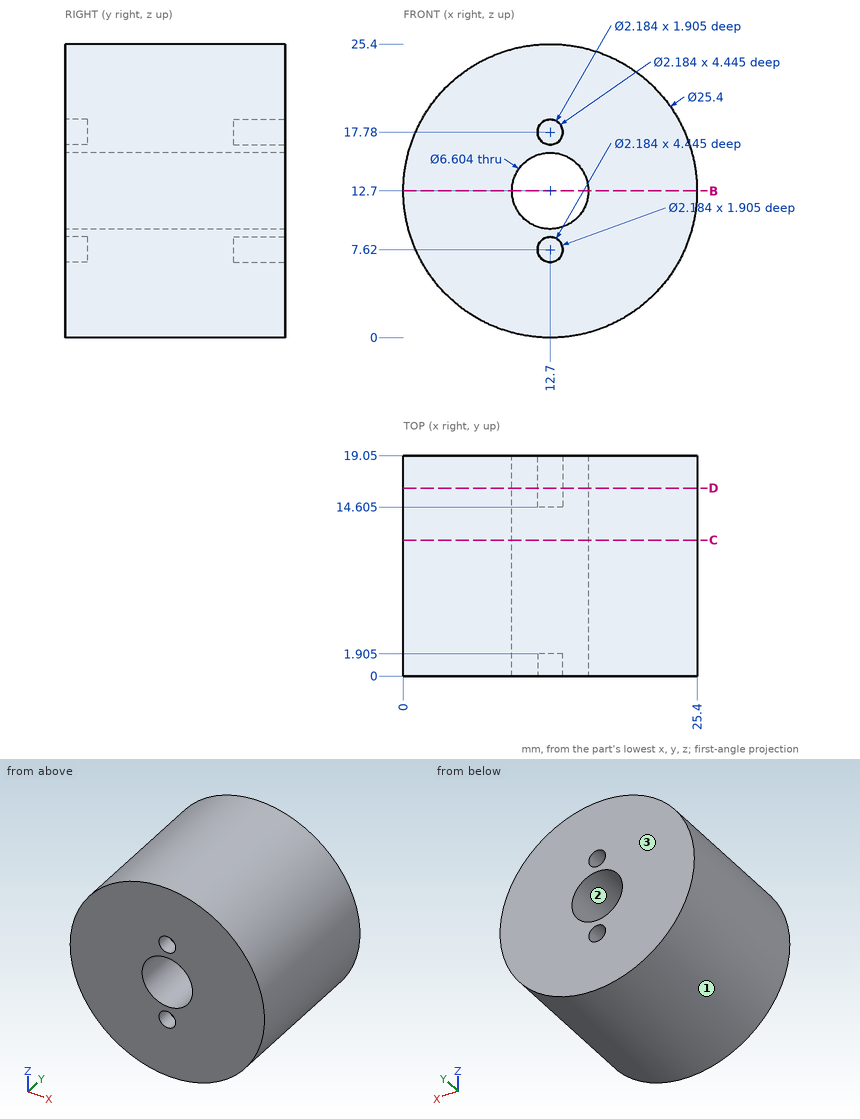
Answer from the drawing. Dimensions are ordinates in mm from the lowest x, y and z of the part. Round coordinates to 2 decimals unless told otherwise and drop trailing zeros. Loops run counter-clockwise (first coordinate to the right, second up) from the corner with the lowest first, then second, coordinate; pieces in that order, holes last. Notation, with made-up numbers: M -12,83 L 2,83 A3 cw 2,88 Z; hole C -14.5,-7 d5. An arc over 180 degrees is marked long. One line per question, with ' | ' between items. Start each with the question number.
(1) A cutting plane is placed at D-D on y = 16.25. Write down the section's boundary in (x, z) (1 decimal).
(2) Flat-ended cylindrical pins translate along their axes: pin 1 Ø0.7 at (x, z) = (13, 18) entering from +Y (3 decimals); pin 2 Ø3 at (x, z) = (4.5, 7.5) entering from -Y; pin 3 Ø10 at (x, y) = (22, 16) entering from -Z; pin 4 Ø2 at (x, z) = (12.7, 17.78) entering from -Y (3 decimals). Find the tip coordinate at first contact, or state that the pin passes through.
(3) A cutting plane is placed at C-C on y = 11.75. Write down the section's boundary in (x, z).
(4) A cutting plane is placed at B-B on z = 12.7. Write down the section's boundary in (x, y).
(5) For a pull along Z with two mould halves and no side action, classify the marked faces 1, 2 and 3 as released by +Z, released by -Z, zero draft, split by the parting line, or undercut.
(6) Find the intervals of material crossed by line 1 (Z direction, x = 12.7, y = 1); line 2 (X direction, y = 0.85, z = 7.62); line 3 (Z direction, x = 15.25, y = 15.25) (1 decimal), in increasing order.
Geometry check:
1) outline: C 12.7,12.7 d25.4; hole C 12.7,12.7 d6.6; hole C 12.7,7.6 d2.2; hole C 12.7,17.8 d2.2
2) pin 1: stops at y = 14.605 | pin 2: stops at y = 0 | pin 3: stops at z = 0.75 | pin 4: stops at y = 1.905
3) outline: C 12.7,12.7 d25.4; hole C 12.7,12.7 d6.6
4) outline: M 0,0 L 9.4,0 L 9.4,19.05 L 0,19.05 Z; M 16,0 L 25.4,0 L 25.4,19.05 L 16,19.05 Z
5) face 1: split by the parting line | face 2: undercut | face 3: zero draft
6) line 1: z = 0 to 6.53, 8.71 to 9.4, 16 to 16.69, 18.87 to 25.4 | line 2: x = 1.06 to 11.61, 13.79 to 24.34 | line 3: z = 0.3 to 10.6, 14.8 to 25.1
